The figure shows three views and two pictorial views of one solid part (mm, origin at its lowest corner). Answer the questions. Coordinates: 2 decimals unless noted, no trailing zeros. Order: outer loops, then holes, each group sorted by start corner. A loop starts at its lowest first (then second) coordinate and runs counter-clockwise, first axis right, second up. Notation, with made-up numbers: (33, -23) -> (45, -23) arc R21 ccw to (45, 7) -> close; hole circle Ø6 at (9, -2.75). An arc over 180 degrees is marked (long way). Write item = value, one per line. Start each with the question number.
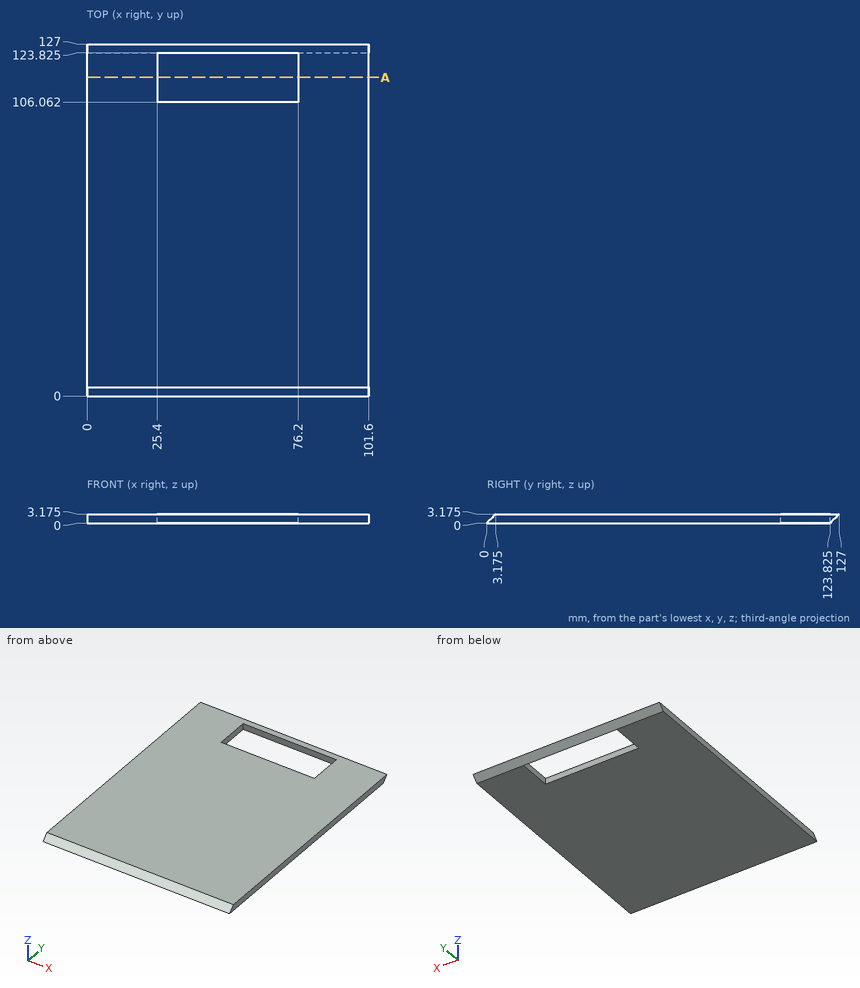
Item 1: Section A-A, the plane y = 115 is taken. Give the vertices of the cut face in (x, z) (1 decimal).
Item 2: This flat-tipped pin is pushed along its axis until it touches: pin 1 (1 mm diameter, centred on x = 58.5, z = 1, fed in from -Y). Where does it stop, or does it pass through?
Item 3: Consider probe 1 along Y at (x, z) = (63, 1.2) (1 decimal); probe 2 along Y at (x, z) = (26.5, 1.8) (1 decimal); probe 3 along Y at (x, z) = (82, 0.6) (1 decimal). Determine where each line is inside the solid, lowest interval first.
A:
q1.outline = (0, 0) -> (25.4, 0) -> (25.4, 3.2) -> (0, 3.2) -> close; (76.2, 0) -> (101.6, 0) -> (101.6, 3.2) -> (76.2, 3.2) -> close
q2.pin_1 = 0.5
q3.probe_1 = 1.2 to 106.1, 123.8 to 125
q3.probe_2 = 1.8 to 106.1, 123.8 to 125.6
q3.probe_3 = 0.6 to 124.4
